Part print with two shaded views. Sizes in mm from the minimum x, y, z corner. A direction names the side the tool comes from. Round coordinates to 2 decimals unless told otherwise and drop trailing zeros. Write each loop counter-clockwise with the first axis right and the second up, starting at its lowest first coordinate (ties: lowest second). Pieces come first, ordered by that corner, then holes. Notation, with made-up numbers: (43, -27) -> (67, -27) arc R24 ccw to (67, 10) -> close; hole circle Ø4 at (67.5, 70). An arc over 180 degrees is marked (long way). Answer in a Markdown table with one row per item.
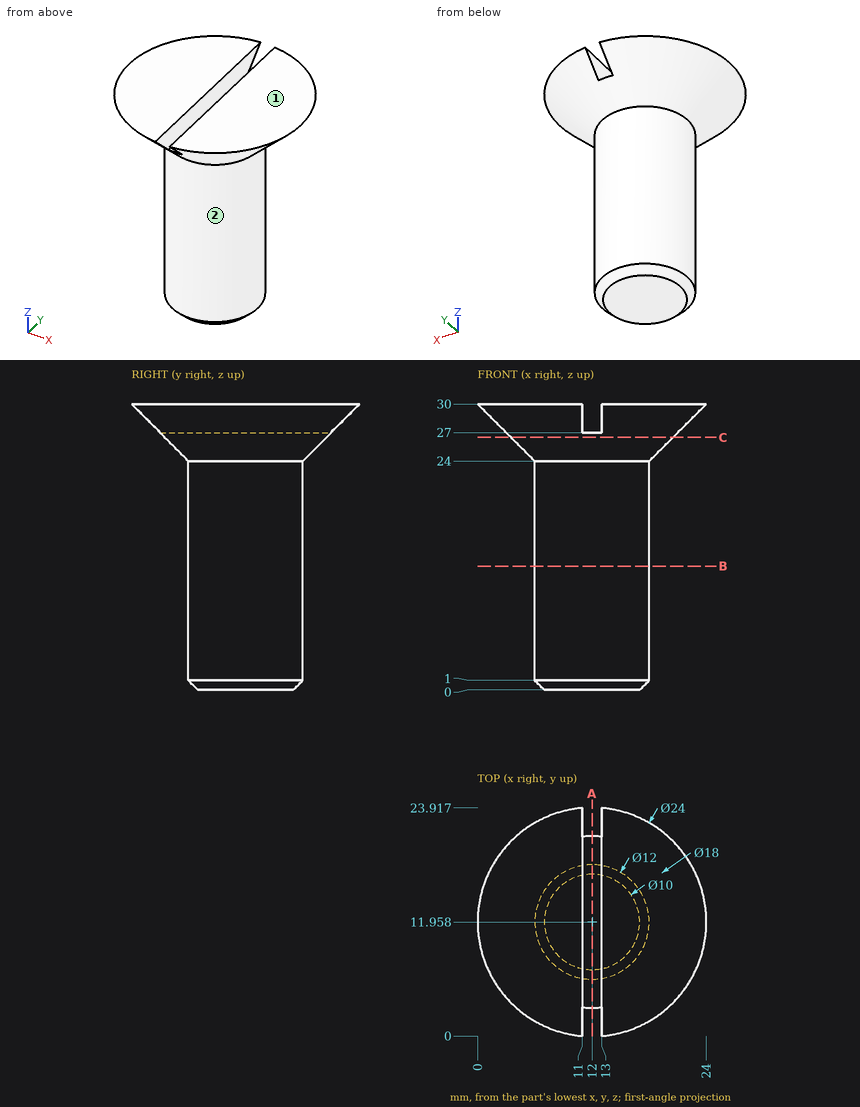
Q1. Saw through at A-A on x = 12. Write the cut outline in (y, z), plus the area to 3 significant figures.
A:
| item | result |
|---|---|
| outline | (2.96, 27) -> (5.96, 24) -> (5.96, 1) -> (6.96, 0) -> (16.96, 0) -> (17.96, 1) -> (17.96, 24) -> (20.96, 27) -> close |
| area | 332 mm² |
Q2. Saw through at B-B on z = 13. Write the cut outline in (x, y).
A:
| item | result |
|---|---|
| outline | circle Ø12 at (12, 11.96) |
Q3. Wall check: line 1 (Z direction, x = 12.5, y = 16); line 2 (X direction, y = 6.5, z = 17.5) (1 decimal); line 3 (Y direction, x = 9, z = 12) (1 decimal). Give the ranges that are in metal, low to high. Write a range as [from, to].
A:
| item | result |
|---|---|
| line 1 | [0, 27] |
| line 2 | [9.5, 14.5] |
| line 3 | [6.8, 17.2] |
Q4. Saw through at C-C on z = 26.5. Write the cut outline in (x, y), plus the area to 3 significant figures.
A:
| item | result |
|---|---|
| outline | circle Ø17 at (12, 11.96) |
| area | 227 mm² |
Q5. Drop flat-ended pins along their axis: P1, Ø2, axis at y = 20.5, z = 22.5, coming from the -X side; P2, Ø6, axis at x = 8.5, z = 16.5, coming from the -Y side; P3, Ø12, axis at y = 11.5, z = 7.5, coming from the -X side; P4, Ø4, axis at x = 5.5, z = 22.5, coming from the -Y side. Give the stop position or say it passes through.
A:
| item | result |
|---|---|
| P1 | through |
| P2 | y = 5.98 |
| P3 | x = 6 |
| P4 | y = 7.99 |
Q6. Which spindle directions (+Z, -Z, +X, -X, +Y, -Y) get a long thin tool onto all of the face, cutting with end or side? Do the marked faces 1 and 2. Say none if no direction does.
A:
| item | result |
|---|---|
| face 1 | +Z, +X, -X, +Y, -Y |
| face 2 | -Z |
